```python
from build123d import *

# Parameters (mm, degrees)
SKETCH1_W              = 69
SKETCH1_H              = 100
BOSS_EXTRUDE1_DEPTH    = 2.5
SKETCH2_W              = 69
SKETCH2_H              = 77
CUT_EXTRUDE1_DEPTH     = 1.2
M2_5_CLEARANCE_HOLE1_D = 3.1


with BuildPart() as part:
    # Sketch1 → Boss-Extrude1 (new body)
    with BuildSketch(Plane(origin=(0, 0, 0), x_dir=(1, 0, 0), z_dir=(0, 1, 0))):
        Rectangle(SKETCH1_W, SKETCH1_H)
    extrude(amount=BOSS_EXTRUDE1_DEPTH)

    # Sketch2 → Cut-Extrude1 (cut)
    with BuildSketch(Plane(origin=(0, 2.5, 0), x_dir=(1, 0, 0), z_dir=(0, 1, 0))):
        Rectangle(SKETCH2_W, SKETCH2_H)
    extrude(amount=-CUT_EXTRUDE1_DEPTH, mode=Mode.SUBTRACT)

    # M2.5 Clearance Hole1 (through all)
    with Locations(Plane(origin=(0, 2.5, 0), x_dir=(1, 0, 0), z_dir=(0, 1, 0))):
        with Locations((-27.5, 45), (27.5, 45), (-27.5, -45), (27.5, -45), (0, 0)):
            Hole(M2_5_CLEARANCE_HOLE1_D / 2)


solid = part.part
```
Geometry: final body of the model. Coordinates: model frame, mm. A direction names the side the tool comes from. Coordinates: 2 decimals unless noted, no trailing zeros. Order: outer loops, then holes, each group sorted by start corner. A loop starts at its lowest first (then second) coordinate and runs counter-clockwise, first axis right, second up.
Item 1: Draft query along X for faces 1 (the face through (0, 1, 50)), 2 (the face through (26.785, 1.233, 46.375)), 3 (the face through (34.5, 1, 1)). Return one class per face: released by +X, released by -X, zero draft, split by the parting line, or undercut.
Answer:
face 1: zero draft
face 2: undercut
face 3: released by +X
Item 2: Section query D-D (z = -45). Output: boundary loops of the cut face in (x, y), then the cut area to 3 significant figures.
Answer:
outline: (-34.5, 0) - (-29.05, 0) - (-29.05, 2.5) - (-34.5, 2.5) - close; (-25.95, 0) - (25.95, 0) - (25.95, 2.5) - (-25.95, 2.5) - close; (29.05, 0) - (34.5, 0) - (34.5, 2.5) - (29.05, 2.5) - close
area: 157 mm2
Item 3: Material intervals for line 1 along Z through (x, y) = (-27.5, 1.6); line 2 along X through (y, z) = (1.55, -45); line 3 along Y through (x, z) = (23.5, 9.5), sorted ascending.
Answer:
line 1: z = -50 to -46.55, -43.45 to -38.5, 38.5 to 43.45, 46.55 to 50
line 2: x = -34.5 to -29.05, -25.95 to 25.95, 29.05 to 34.5
line 3: y = 0 to 1.3
Item 4: Access query for faces 4 (the face through (-0.715, 0.641, 1.375)), 5 (the face through (7, 1.3, -1)). Directions: +Z, -Z, +X, -X, +Y, -Y. A direction counts if a zero-diameter tool reaches every point of the face in a straight line with its end or side. Return the directions, or none.
Answer:
face 4: +Y, -Y
face 5: +X, -X, +Y
Item 5: Section query A-A (y = 1.75). Output: boundary loops of the cut face in (x, z).
Answer:
outline: (-34.5, -50) - (34.5, -50) - (34.5, -38.5) - (-34.5, -38.5) - close; (-34.5, 38.5) - (34.5, 38.5) - (34.5, 50) - (-34.5, 50) - close; hole circle Ø3.1 at (-27.5, -45); hole circle Ø3.1 at (-27.5, 45); hole circle Ø3.1 at (27.5, -45); hole circle Ø3.1 at (27.5, 45)
Item 6: Contact query for a flat-ended pin moving along its axis: P1, Ø2.5, axis at x = -27.5, z = -45, coming from the -Y side. Output: stop coordinate, or through.
Answer:
P1: passes through
Item 7: Section query C-C (x = -27.5). Output: boundary loops of the cut face in (y, z), then the cut area to 3 significant figures.
Answer:
outline: (0, -50) - (2.5, -50) - (2.5, -46.55) - (0, -46.55) - close; (0, -43.45) - (2.5, -43.45) - (2.5, -38.5) - (1.3, -38.5) - (1.3, 38.5) - (2.5, 38.5) - (2.5, 43.45) - (0, 43.45) - close; (0, 46.55) - (2.5, 46.55) - (2.5, 50) - (0, 50) - close
area: 142 mm2
Item 8: Section query B-B (z = 0). Output: boundary loops of the cut face in (x, y), then the cut area to 3 significant figures.
Answer:
outline: (-34.5, 0) - (-1.55, 0) - (-1.55, 1.3) - (-34.5, 1.3) - close; (1.55, 0) - (34.5, 0) - (34.5, 1.3) - (1.55, 1.3) - close
area: 85.7 mm2
